Verification items for this drawing (mm, ordinates from the low corner). A direction names the side the tool comes from. Give positions to 0.01 mm unless a question says otherwise; leave off trailing zeros. Order: outer loops, then holes, each group sorted by start corner. A loop starts at its lowest first (then second) coordinate and runs counter-clockwise, first axis right, second up.
(1) Gauge pin test, flat ends, axial feed: pin 1 (2 mm diameter, centred on y = 10, z = 3.5, fed in from -X); pin 2 (1.5 mm diameter, centred on x = 12, y = 8.5, fed in from +Z). Record the tip position at first contact, or that the pin passes through.
(2) Scan lines: L1, parallel to Y at x = 4.5, z = 5.75; L2, parallel to Z at x = 1, y = 7.5; L3, parallel to X at y = 11, z = 6.75. Record each from-to range of solid material in increasing order.
(3) Sectioned sample at A-A on z = 6.5. Record the cut outline in (x, y).
(4) Sectioned sample at D-D on y = 5.5. Record the cut outline in (x, z).
(5) Sectioned sample at B-B on x = 7. Record the cut outline in (y, z), plus the area to 3 significant figures.
(6) Sectioned sample at C-C on y = 10.5. Record the cut outline in (x, z), plus the area to 3 significant figures.
(7) Access from +Z, -Z, +X, -X, +Y, -Y to the whole of each face (thin tool, end or side, straight path). Record for the marked faces 5, 6 and 7.
(8) Mould release check, pull along Y, two halves, no side actions. Record for the marked faces 1, 2, 3 and 4: pulls with the +Y half, pulls with the -Y half, needs draft (parallel to the pull), parting line crosses it, or undercut.
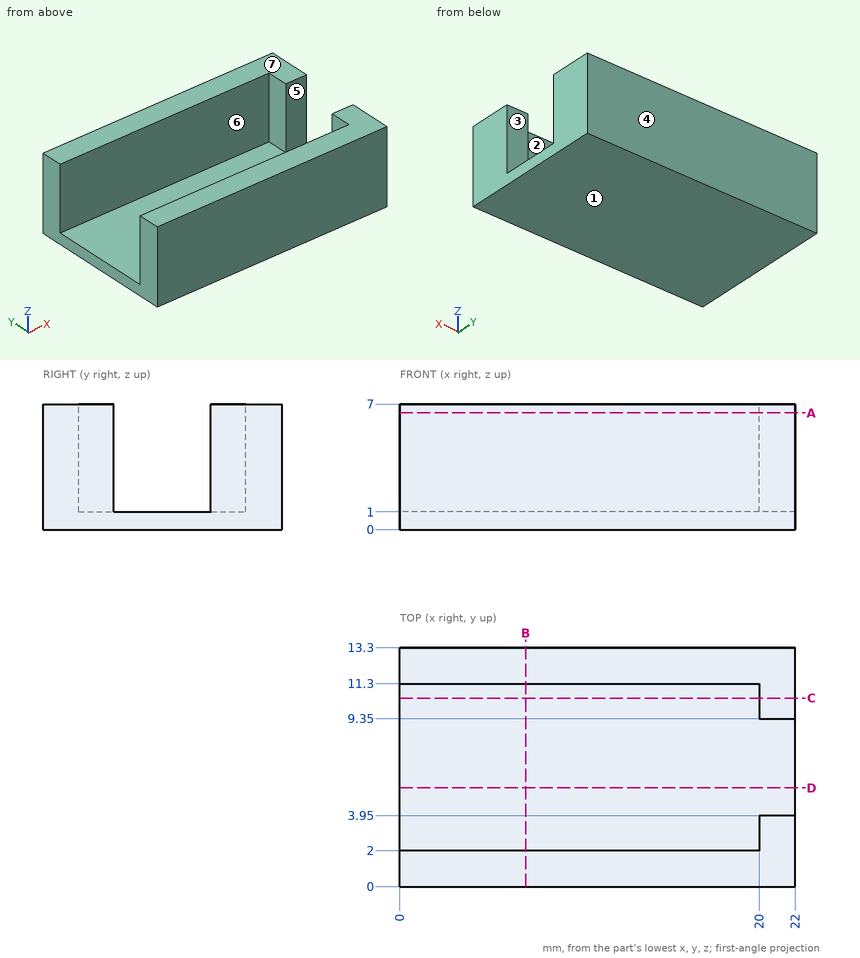
Ans:
1. pin 1: stops at x = 20
1. pin 2: stops at z = 1
2. L1: y = 0 to 2, 11.3 to 13.3
2. L2: z = 0 to 1
2. L3: x = 20 to 22
3. outline: (0, 0) - (22, 0) - (22, 3.95) - (20, 3.95) - (20, 2) - (0, 2) - close; (0, 11.3) - (20, 11.3) - (20, 9.35) - (22, 9.35) - (22, 13.3) - (0, 13.3) - close
4. outline: (0, 0) - (22, 0) - (22, 1) - (0, 1) - close
5. outline: (0, 0) - (13.3, 0) - (13.3, 7) - (11.3, 7) - (11.3, 1) - (2, 1) - (2, 7) - (0, 7) - close
5. area: 37.3 mm2
6. outline: (0, 0) - (22, 0) - (22, 7) - (20, 7) - (20, 1) - (0, 1) - close
6. area: 34.0 mm2
7. face 5: +Z, +X, -X
7. face 6: +Z, -X
7. face 7: +Z, +X, -X, +Y, -Y
8. face 1: needs draft
8. face 2: undercut
8. face 3: undercut
8. face 4: pulls with the +Y half
